Design review of the part built by this model. Coordinates are the model's own, in mm. A direction names the side the tool comes from. Round coordinates to 2 decimals unless told otherwise and drop trailing zeros. Loops run counter-clockwise (first coordinate to the right, second up) from the corner with the lowest first, then second, coordinate; pieces in that order, holes last. Notation, with made-up numbers: M 41,29 L 55,29 A12 cw 55,33 Z; hole C 77,70 d2. An arc over 180 degrees is marked long. Use a Markdown table: item, result.
from build123d import *

# Parameters (mm, degrees)
ESBO_O1_W                         = 30
ESBO_O1_H                         = 30
RESSALTO_EXTRUS_O1_DEPTH          = 50
CORTE_EXTRUS_O1_START             = -5
ESBO_O2_W                         = 25
ESBO_O2_H                         = 5
CORTE_EXTRUS_O1_DEPTH             = 26
CORTE_EXTRUS_O2_START             = -5
ESBO_O3_W                         = 25
ESBO_O3_H                         = 25
CORTE_EXTRUS_O2_DEPTH             = 26
FURO_COM_FOLGA_DE_M41_D           = 4.5
FURO_COM_FOLGA_DE_M41_ON_FACE_2_D = 4.5


with BuildPart() as part:
    # Esboço1 → Ressalto-extrusão1 (new body)
    with BuildSketch(Plane.XY):
        with Locations((-15, 15)):
            Rectangle(ESBO_O1_W, ESBO_O1_H)
    extrude(amount=RESSALTO_EXTRUS_O1_DEPTH)

    # Esboço2 → Corte-extrusão1 (cut, through all)
    with BuildSketch(Plane(origin=(0, 30, 0), x_dir=(1, 0, 0), z_dir=(0, 1, 0)).offset(CORTE_EXTRUS_O1_START)):
        with Locations((-17.5, -12.5)):
            Rectangle(ESBO_O2_W, ESBO_O2_H)
    extrude(amount=-CORTE_EXTRUS_O1_DEPTH, mode=Mode.SUBTRACT)

    # Esboço3 → Corte-extrusão2 (cut, through all)
    with BuildSketch(Plane(origin=(0, 30, 0), x_dir=(1, 0, 0), z_dir=(0, 1, 0)).offset(CORTE_EXTRUS_O2_START)):
        with Locations((-17.5, -37.5)):
            Rectangle(ESBO_O3_W, ESBO_O3_H)
    extrude(amount=-CORTE_EXTRUS_O2_DEPTH, mode=Mode.SUBTRACT)

    # Furo com folga de M41 (through all)
    with Locations(Plane(origin=(-5, 15, 35), x_dir=(0, 0, -1), z_dir=(-1, 0, 0))):
        with Locations((0, 0)):
            Hole(FURO_COM_FOLGA_DE_M41_D / 2)

    # Furo com folga de M41 on face 2 (through all)
    with Locations(Plane(origin=(-15, 25, 35), x_dir=(0, 0, -1), z_dir=(0, -1, 0))):
        with Locations((0, 0)):
            Hole(FURO_COM_FOLGA_DE_M41_ON_FACE_2_D / 2)


solid = part.part
1. Take a section at B-B on y = 15. Give the boundary of the cut face in (x, z), and give its area (4 significant figures).
Check values:
| item | result |
|---|---|
| outline | M -30,0 L 0,0 L 0,32.75 L -5,32.75 L -5,25 L -30,25 L -30,15 L -5,15 L -5,10 L -30,10 Z; M -5,37.25 L 0,37.25 L 0,50 L -5,50 Z |
| area | 727.5 mm² |
2. Take a section at D-D on y = 21.5. Give the boundary of the cut face in (x, z), and give its area (3 significant figures).
Check values:
| item | result |
|---|---|
| outline | M -30,0 L 0,0 L 0,50 L -5,50 L -5,25 L -30,25 L -30,15 L -5,15 L -5,10 L -30,10 Z |
| area | 750 mm² |
3. Take a section at A-A on x = -15. Give the boundary of the cut face in (y, z).
Check values:
| item | result |
|---|---|
| outline | M 0,0 L 30,0 L 30,32.75 L 25,32.75 L 25,25 L 0,25 L 0,15 L 25,15 L 25,10 L 0,10 Z; M 25,37.25 L 30,37.25 L 30,50 L 25,50 Z |
4. Wall thickness on line 1 along Y through (x, z) = (-3.55, 35); line 2 along X through (y, z) = (28.25, 35); line 3 along Z through (x, y) = (-12.25, 11): over which ranges is each line inside the solid? List them lowest first. Write a range as from..to.
Check values:
| item | result |
|---|---|
| line 1 | y = 0..12.75, 17.25..30 |
| line 2 | x = -30..-17.25, -12.75..0 |
| line 3 | z = 0..10, 15..25 |
5. Take a section at C-C on z = 35. Give the boundary of the cut face in (x, y).
Check values:
| item | result |
|---|---|
| outline | M -30,25 L -17.25,25 L -17.25,30 L -30,30 Z; M -12.75,25 L -5,25 L -5,17.25 L 0,17.25 L 0,30 L -12.75,30 Z; M -5,0 L 0,0 L 0,12.75 L -5,12.75 Z |
6. Insertion check: pin 1 (1.5 mm diameter, centred on y = 8.5, z = 12, fed in from -X); pin 2 (6 mm diameter, centred on x = -15, z = 35, fed in from -Y). Each pin has a flat end and moves straight along its axis. Give the tip position at first contact, or say it passes through.
Check values:
| item | result |
|---|---|
| pin 1 | stops at x = -5 |
| pin 2 | stops at y = 25 |
7. The part is to be moulded in two halves that separate along Y. For faces 4 (the face through (-2.47, 15.86, 37.08)), 5 (the face through (-18, 13, 10)), 6 (the face through (-15, 30, 25)), 7 (the face through (-15, 0, 19)), say which applies: pulls with the +Y half, pulls with the -Y half, needs draft (parallel to the pull), parting line crosses it, or undercut.
Check values:
| item | result |
|---|---|
| face 4 | undercut |
| face 5 | needs draft |
| face 6 | pulls with the +Y half |
| face 7 | pulls with the -Y half |
8. Machinability: for faces 1 (the face through (-15.86, 27.53, 37.08)), 2 (the face through (-18, 13, 15)), 3 (the face through (-18, 13, 25)), which of the approach directions +Z, -Z, +X, -X, +Y, -Y give a long, thin tool a straight path to every point of the face, cutting with its end or side? Answer none if there is none.
Check values:
| item | result |
|---|---|
| face 1 | +Y, -Y |
| face 2 | -X, -Y |
| face 3 | +Z, -X, -Y |
